```python
from build123d import *


with BuildPart() as f1:
    # F0 (on Front) → F1 (revolve)
    with BuildSketch(Plane.XZ):
        with BuildLine():
            Line((-48.432033, -5.520982), (-48.432033, -43.520982))
            ThreePointArc((-48.432033, -43.520982), (-46.967567, -47.056516), (-43.432033, -48.520982))
            Line((-43.432033, -48.520982), (-43.432033, -43.520982))
            Line((-43.432033, -43.520982), (-43.432033, 22.979018))
            Line((-43.432033, 22.979018), (-43.432033, 25.479018))
            Line((-43.432033, 25.479018), (-43.432033, 41.479018))
            Line((-43.432033, 41.479018), (-45.932045, 41.479018))
            Line((-45.932045, 41.479018), (-45.932045, 25.479018))
            Line((-45.932045, 25.479018), (-48.432045, 25.479018))
            Line((-48.432045, 25.479018), (-48.432045, 22.979018))
            ThreePointArc((-48.432045, 22.979018), (-46.634149, 22.276914), (-45.932045, 20.479018))
            Line((-45.932045, 20.479018), (-46.932033, -4.020982))
            ThreePointArc((-46.932033, -4.020982), (-47.389147, -5.063868), (-48.432033, -5.520982))
        make_face()
    revolve(axis=Axis((-43.432033, 0, -10.270982), (0, 0, 1)))


solid = f1.part
```
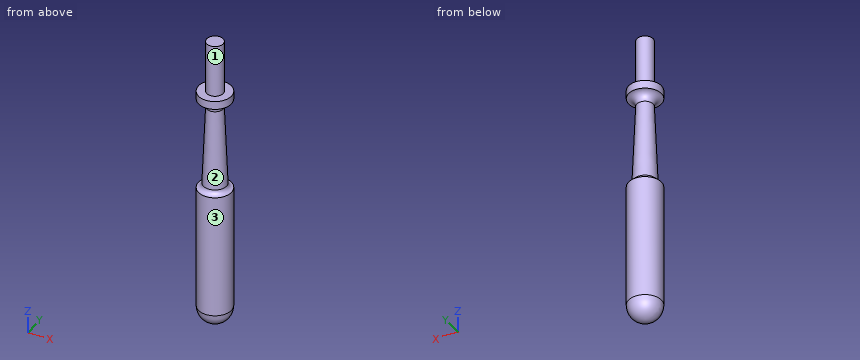
Verification items for the finished model (mm, model axes). Face numbers are marked on the shaded views. A direction names the side the tool comes from. Coordinates: 2 decimals unless noted, no trailing zeros. Loops run counter-clockwise (first coordinate to the right, second up) from the corner with the lowest first, then second, coordinate; pieces in that order, holes last. Notation, with made-up numbers: (-9, 1.5) - (45, 1.5) arc R32 cw to (45, 35.5) - close; hole circle Ø1 at (53, 51). An arc over 180 degrees is marked (long way). Answer as a JSON object with one key per item and string values.
(1) Scan lines: line 1 along Z through (x, y) = (-47.25, 0.5); line 2 along Z through (x, y) = (-39.75, 2.25); line 3 along X through (y, z) = (-3, -5). Record each from-to range of solid material in increasing order.
Response:
{"line 1": "z = -46.71 to -4.95, 22.74 to 25.48", "line 2": "z = -46.05 to -5.33, 22.91 to 25.48", "line 3": "x = -45.92 to -40.95"}
(2) Cross-section at B-B, the plane z = 15. Record the boundary of the cut face in (x, y).
Response:
{"outline": "circle Ø5.45 at (-43.43, 0)"}
(3) Access from +Z, -Z, +X, -X, +Y, -Y to the whole of each face (thin tool, end or side, straight path). Record for the marked faces 1, 2 and 3.
Response:
{"face 1": "+Z", "face 2": "none", "face 3": "+Z, -Z"}
(4) Cross-section at A-A, the plane z = -16. Record the boundary of the cut face in (x, y).
Response:
{"outline": "circle Ø10 at (-43.43, 0)"}
(5) Go/stop test with flat-tipped pins: pin 1 Ø2 at (x, y) = (-42.5, 2) entering from -Z; pin 2 Ø4 at (y, z) = (-1, 9.5) entering from +X; pin 3 Ø1.5 at (y, z) = (1.5, 12) entering from -X. Record where each tip stops, or that it passes through.
Response:
{"pin 1": "stops at z = -48.37", "pin 2": "stops at x = -40.41", "pin 3": "stops at x = -46.18"}
